from build123d import *

# Parameters (mm, degrees)
SKETCH1_R           = 2.286
SKETCH1_R_2         = 2.54
BOSS_EXTRUDE1_DEPTH = 12.573
SKETCH2_W           = 38.1
SKETCH2_H           = 12.954
CUT_EXTRUDE1_DEPTH  = 37.433951597
SKETCH3_R           = 4.445
CUT_EXTRUDE2_DEPTH  = 2.54
BOSS_EXTRUDE2_START = -6.096
SKETCH4_R           = 2.286
SKETCH4_R_2         = 1.905
BOSS_EXTRUDE2_DEPTH = 6.096
FILLET1_R           = 3.81
SKETCH6_W           = 12.7
SKETCH6_H           = 8.255
CUT_EXTRUDE4_DEPTH  = 37.433951597
FILLET2_R           = 1.27


with BuildPart() as part:
    # Sketch1 → Boss-Extrude1 (new, symmetric)
    with BuildSketch(Plane(origin=(0, 0, 0), x_dir=(1, 0, 0), z_dir=(0, 1, 0))):
        with BuildLine():
            Line((-25.4, 6.35), (25.4, 6.35))
            ThreePointArc((25.4, 6.35), (31.75, 0), (25.4, -6.35))
            Line((25.4, -6.35), (-25.4, -6.35))
            ThreePointArc((-25.4, -6.35), (-31.75, 0), (-25.4, 6.35))
        make_face()
        with Locations(Location((-25.4, 0, 0), (0, 0, 270))):
            Circle(SKETCH1_R, mode=Mode.SUBTRACT)
        with Locations(Location((25.4, 0, 0), (0, 0, 270))):
            Circle(SKETCH1_R_2, mode=Mode.SUBTRACT)
    extrude(amount=BOSS_EXTRUDE1_DEPTH, both=True)

    # Sketch2 → Cut-Extrude1 (cut, through all)
    with BuildSketch(Plane.XY.offset(6.35)):
        with Locations((-12.7, 0)):
            Rectangle(SKETCH2_W, SKETCH2_H)
    extrude(amount=-CUT_EXTRUDE1_DEPTH, mode=Mode.SUBTRACT)

    # Sketch3 → Cut-Extrude2 (cut)
    with BuildSketch(Plane(origin=(0, 12.573, 0), x_dir=(1, 0, 0), z_dir=(0, 1, 0))):
        with Locations(Location((-25.4, 0, 0), (0, 0, 270))):
            Circle(SKETCH3_R)
    extrude(amount=-CUT_EXTRUDE2_DEPTH, mode=Mode.SUBTRACT)

    # Sketch4 → Boss-Extrude2 (add)
    with BuildSketch(Plane(origin=(0, -6.477, 0), x_dir=(1, 0, 0), z_dir=(0, 1, 0)).offset(BOSS_EXTRUDE2_START)):
        with Locations(Location((-25.4, 0, 0), (0, 0, 270))):
            Circle(SKETCH4_R)
        with Locations(Location((-25.4, 0, 0), (0, 0, 180))):
            Circle(SKETCH4_R_2, mode=Mode.SUBTRACT)
    extrude(amount=BOSS_EXTRUDE2_DEPTH)

    # Fillet1
    fillet1_edges = [part.edges().sort_by_distance(p)[0] for p in [
        (6.35, 0, 6.35),
        (6.35, 0, -6.35),
    ]]
    fillet(fillet1_edges, radius=FILLET1_R)

    # Sketch6 → Cut-Extrude4 (cut, through all)
    with BuildSketch(Plane.XY.offset(6.35)):
        with Locations((25.4, -5.9055)):
            Rectangle(SKETCH6_W, SKETCH6_H)
    extrude(amount=-CUT_EXTRUDE4_DEPTH, mode=Mode.SUBTRACT)

    # Fillet2
    fillet2_edges = [part.edges().sort_by_distance(p)[0] for p in [
        (19.05, -5.9055, 6.35),
        (19.05, -5.9055, -6.35),
    ]]
    fillet(fillet2_edges, radius=FILLET2_R)


solid = part.part
Geometry: final body of the model. Coordinates: model frame, mm. A direction names the side the tool comes from. Give positions to 0.01 mm unless a question says otherwise; leave off trailing zeros. Loops run counter-clockwise (first coordinate to the right, second up) from the corner with the lowest first, then second, coordinate; pieces in that order, holes last. Notation, with made-up numbers: M 12.5,-21 L 33.5,-21 A22 cw 33.5,7 Z; hole C 4,68 d11. An arc over 180 degrees is marked long. Put each result on its own line as item: value.
1) Reachability of faces 1 (the flat face through (6.35, 0, 0)), 2 (the cylindrical face through (7.496, 0.091, 5.264)), 3 (the flat face through (19.05, -6, 0)), 4 (the flat face through (-23, 10.033, -1)) from +Z, -Z, +X, -X, +Y, -Y: full face, straight path, thin tool, end or side. Return the list, or none.
Computed values:
face 1: +Z, -Z, -X
face 2: +Z, -X
face 3: +Z, -Z, +X
face 4: +Y
2) Cut plane A-A, the plane z = 0. Give the number of separate pieces and of enclosed holes in the cut face, plus the area to 3 significant figures.
Computed values:
separate pieces: 5
enclosed holes: 0
area: 851 mm^2
3) Cut plane B-B, the plane x = -2. Return the cut outline in (y, z), plus the area to 3 significant figures.
Computed values:
outline: M -12.57,-6.35 L -6.48,-6.35 L -6.48,6.35 L -12.57,6.35 Z; M 6.48,-6.35 L 12.57,-6.35 L 12.57,6.35 L 6.48,6.35 Z
area: 155 mm^2
4) Material intervals for L1, parallel to X at y = 8, z = -0.25; L2, parallel to Z at x = -25.4, y = 8.75; L3, parallel to Y at x = -26, z = -4, sorted ascending. Write a range as from..to.
Computed values:
L1: x = -31.75..-27.67, -23.13..22.87, 27.93..31.75
L2: z = -6.35..-2.29, 2.29..6.35
L3: y = -12.57..-6.48, 6.48..10.03
5) Cut plane D-D, the plane y = 7.75. Return the cut outline in (x, z).
Computed values:
outline: M -25.4,-6.35 L 25.4,-6.35 A6.35 ccw 25.4,6.35 L -25.4,6.35 A6.35 ccw Z; hole C -25.4,0 d4.57; hole C 25.4,0 d5.08
6) Mould query, pull axis Z, two halves, no side actions, for faces 5 (the cylindrical face through (7.496, 0.091, -5.264)), 6 (the cylindrical face through (18.688, -5.848, 5.968)), 7 (the cylindrical face through (31.75, 5.5, -0.14)), 8 (the cylindrical face through (-23.133, 8.23, -0.298)). Classes: released by +Z, released by -Z, zero draft, split by the parting line, or undercut.
Computed values:
face 5: released by -Z
face 6: released by +Z
face 7: split by the parting line
face 8: undercut
7) Cut plane C-C, the plane y = 1. Return the cut outline in (x, z), plus the area to 3 significant figures.
Computed values:
outline: M 6.35,-2.54 A3.81 ccw 10.16,-6.35 L 25.4,-6.35 A6.35 ccw 25.4,6.35 L 10.16,6.35 A3.81 ccw 6.35,2.54 Z; hole C 25.4,0 d5.08
area: 279 mm^2
8) First-contact query: P1, Ø4, axis at x = -25.4, z = 0, coming from the +Y side; P2, Ø4, axis at y = 0.5, z = 1, coming from the -X side; P3, Ø5, axis at y = -5, z = 5, coming from the +X side; P4, Ø4.5, axis at x = 25.4, z = 0, coming from the -Y side. Flat tips, straight axial feed; report the tip coordinate or a pass-through.
Computed values:
P1: stops at y = -6.48
P2: stops at x = 6.35
P3: stops at x = 19.05
P4: passes through
